from build123d import *

# Parameters (mm, degrees)
F1_DEPTH = 40
F2_W     = 20
F2_H     = 20
F3_DEPTH = 20
F4_R     = 10
F5_DEPTH = 20


with BuildPart() as f1:
    # F0 (on Front) → F1 (new body)
    with BuildSketch(Plane.XZ):
        Polygon((-26.586315, 18.18695), (-36.586315, 18.18695), (-36.586315, -21.81305), (33.413685, -21.81305), (33.413685, -1.81305), (-6.586315, -1.81305), align=None)
        Polygon((-6.586315, 18.18695), (-26.586315, 18.18695), (-6.586315, -1.81305), align=None)
    extrude(amount=F1_DEPTH)

    # F2 (on face) → F3 (cut)
    with BuildSketch(Plane.XY.offset(18.18695)):
        with Locations((-16.586315, -20)):
            Rectangle(F2_W, F2_H)
    extrude(amount=-F3_DEPTH, mode=Mode.SUBTRACT)

    # F4 (on face) → F5 (cut)
    with BuildSketch(Plane.XY.offset(-1.81305)):
        with Locations((13.413685, -20)):
            Circle(F4_R)
    extrude(amount=-F5_DEPTH, mode=Mode.SUBTRACT)


solid = f1.part
Verification items for the finished model (mm, model axes). A direction names the side the tool comes from. Round coordinates to 2 decimals unless told otherwise and drop trailing zeros. Order: outer loops, then holes, each group sorted by start corner. A loop starts at its lowest first (then second) coordinate and runs counter-clockwise, first axis right, second up.
1. Section check B-B on x = -22. Record the cut outline in (y, z), then the cut area to 3 significant figures.
Final values:
outline: (-40, -21.81) - (0, -21.81) - (0, 18.19) - (-10, 18.19) - (-10, -1.81) - (-30, -1.81) - (-30, 18.19) - (-40, 18.19) - close
area: 1,200 mm2
2. Go/stop test with flat-tipped pins: P1, Ø10, axis at y = -17.5, z = 8, coming from the +X side; P2, Ø8, axis at y = -35, z = 3.5, coming from the +X side. Record where each tip stops, or that it passes through.
Final values:
P1: stops at x = -26.59
P2: stops at x = -6.59
3. Access from +Z, -Z, +X, -X, +Y, -Y to the whole of each face (thin tool, end or side, straight path). Record for faces 1 (the flat face through (-6.586, -35, 8)), 2 (the flat face through (-28, -20, 18.187)), 3 (the flat face through (-17, -30, 8)).
Final values:
face 1: +Z, +X, +Y, -Y
face 2: +Z, +X, -X, +Y, -Y
face 3: +Z, +X
4. Section check A-A on y = -20. Record the cut outline in (x, z).
Final values:
outline: (-36.59, -21.81) - (3.41, -21.81) - (3.41, -1.81) - (-26.59, -1.81) - (-26.59, 18.19) - (-36.59, 18.19) - close; (23.41, -21.81) - (33.41, -21.81) - (33.41, -1.81) - (23.41, -1.81) - close
5. Section check C-C on z = 9. Record the cut outline in (x, y), then the cut area to 3 significant figures.
Final values:
outline: (-36.59, -40) - (-6.59, -40) - (-6.59, -30) - (-26.59, -30) - (-26.59, -10) - (-6.59, -10) - (-6.59, 0) - (-36.59, 0) - close
area: 800 mm2
6. Thickness scan on L1, parallel to Y at x = -20, z = 0; L2, parallel to Z at x = -6.5, y = -27; L3, parallel to X at y = -25, z = 6. Record the ranges inside material, lowest first.
Final values:
L1: y = -40 to -30, -10 to 0
L2: z = -21.81 to -1.81
L3: x = -36.59 to -26.59
7. Section check D-D on z = -15. Record the cut outline in (x, y).
Final values:
outline: (-36.59, -40) - (33.41, -40) - (33.41, 0) - (-36.59, 0) - close; hole circle Ø20 at (13.41, -20)
